```python
from build123d import *

# Parameters (mm, degrees)
SKETCH040_R     = 2.38125
PAD011_DEPTH    = 50.8
CHAMFER_SIZE    = 1
CHAMFER001_SIZE = 1


with BuildPart() as part:
    # Sketch040 → Pad011 (new body)
    with BuildSketch(Plane.XZ):
        Circle(SKETCH040_R)
    extrude(amount=PAD011_DEPTH)

    # Chamfer
    chamfer_edges = [part.edges().sort_by_distance(p)[0] for p in [
        (-2.38125, -50.8, 0),
    ]]
    chamfer(chamfer_edges, length=CHAMFER_SIZE)

    # Chamfer001
    chamfer001_edges = [part.edges().sort_by_distance(p)[0] for p in [
        (-2.38125, 0, 0),
    ]]
    chamfer(chamfer001_edges, length=CHAMFER001_SIZE)


solid = part.part
```
Can you work these out from the model? Positions are in its coordinate system, mm. Round coordinates to 2 decimals unless told otherwise and drop trailing zeros. Loops run counter-clockwise (first coordinate to the right, second up) from the corner with the lowest first, then second, coordinate; pieces in that order, holes last.
Item 1: Will this pin go through, and if not, where does the flat tip stop? pin 1 Ø2 at (x, y) = (-1.5, -31) entering from +Z.
Item 2: Please list where these lines run through material, in increasing order: L1, parallel to Z at x = -0.1, y = -10; L2, parallel to Z at x = 1.3, y = -32.
Item 3: Suppose I cut it at A-A, the plane y = -28.5. Write out the boundary of the cut face in (x, z).
Reported:
1. pin 1: stops at z = 2.33
2. L1: z = -2.38 to 2.38
2. L2: z = -2 to 2
3. outline: circle Ø4.76 at (0, 0)
